```python
from build123d import *

# Parameters (mm, degrees)
ESQUISSE1_R        = 2
ESQUISSE1_W        = 5
ESQUISSE1_H        = 5
BOSS_EXTRU_1_DEPTH = 5
CONG_1_R           = 2


with BuildPart() as part:
    # Esquisse1 → Boss.-Extru.1 (new body)
    with BuildSketch(Plane.XY):
        with BuildLine():
            Line((-72.827296486, -27.9), (-72.827296486, 27.9))
            Line((-72.827296486, 27.9), (-25.4, 27.9))
            ThreePointArc((-25.4, 27.9), (-7.439487758, 20.460512242), (0, 2.5))
            Line((0, 2.5), (-10, 2.5))
            ThreePointArc((-10, 2.5), (-13.202056301, 3.42586604), (-15.41588754, 5.917721519))
            ThreePointArc((-15.41588754, 5.917721519), (-41.577296486, 0), (-15.41588754, -5.917721519))
            ThreePointArc((-15.41588754, -5.917721519), (-13.202056301, -3.42586604), (-10, -2.5))
            Line((-10, -2.5), (0, -2.5))
            ThreePointArc((0, -2.5), (-7.439487758, -20.460512242), (-25.4, -27.9))
            Line((-25.4, -27.9), (-72.827296486, -27.9))
        make_face()
        with Locations((-62.827296486, 0)):
            Circle(ESQUISSE1_R, mode=Mode.SUBTRACT)
        with Locations((-27.827296486, 20.4)):
            Rectangle(ESQUISSE1_W, ESQUISSE1_H, mode=Mode.SUBTRACT)
        Polygon((-9.245314739, 13.615063509), (-6.745314739, 9.284936491), (-11.075441758, 6.784936491), (-13.575441758, 11.115063509), align=None, mode=Mode.SUBTRACT)
        Polygon((-6.745314739, -9.284936491), (-9.245314739, -13.615063509), (-13.575441758, -11.115063509), (-11.075441758, -6.784936491), align=None, mode=Mode.SUBTRACT)
        with Locations((-27.827296486, -20.4)):
            Rectangle(ESQUISSE1_W, ESQUISSE1_H, mode=Mode.SUBTRACT)
        Polygon((-46.409278233, -13.615063509), (-48.909278233, -9.284936491), (-44.579151214, -6.784936491), (-42.079151214, -11.115063509), align=None, mode=Mode.SUBTRACT)
        Polygon((-48.909278233, 9.284936491), (-46.409278233, 13.615063509), (-42.079151214, 11.115063509), (-44.579151214, 6.784936491), align=None, mode=Mode.SUBTRACT)
    extrude(amount=BOSS_EXTRU_1_DEPTH)

    # Congé1
    cong_1_edges = [part.edges().sort_by_distance(p)[0] for p in [
        (0, 2.5, 2.5),
        (0, -2.5, 2.5),
    ]]
    fillet(cong_1_edges, radius=CONG_1_R)


solid = part.part
```
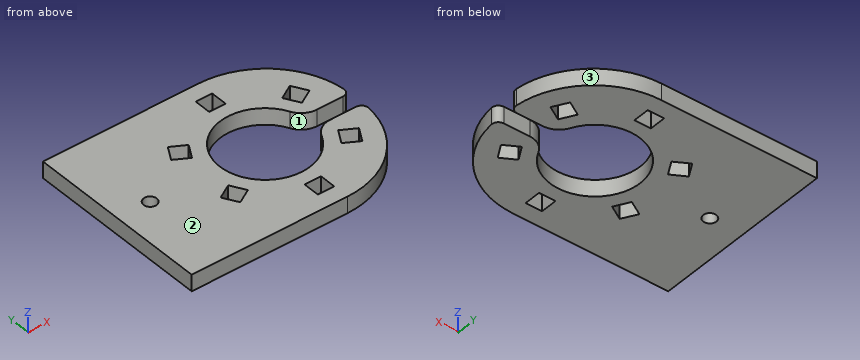
Source: CAD feature listing. Evaluate the final solid. Frame: model axes, mm. Face numbers are marked on the shaded views. Give positions to 0.01 mm unless a question says otherwise; leave off trailing zeros. Write each loop counter-clockwise with the first axis right and the second up, starting at its lowest first coordinate (ties: lowest second). Pieces come first, ordered by that corner, then holes.
1. First-contact query: pin 1 (3 mm diameter, centred on x = -62.83, y = 0, fed in from +Z); pin 2 (2.5 mm diameter, centred on x = -6, z = 2, fed in from +Y); pin 3 (1.5 mm diameter, centred on x = -7.5, z = 2, fed in from -Y); pin 4 (1.5 mm diameter, centred on y = -20, z = 2, fed in from +X). Flat tips, straight axial feed; report the tip coordinate or a pass-through.
2. Pull-direction query (X, two-part tool) for the marked faces 1, 2 and 3; classes: +X half, -X half, draft (parallel to the pull), parting line (faces both ways), or undercut.
3. Section query C-C (y = 24). Return the cut outline in (x, z), then the cut area to 3 significant figures.
4. Material intervals for line 1 along X through (y, z) = (12, 4.15); line 2 along Y through (x, z) = (-10, 2.9); line 3 along X through (y, z) = (-10, 2.3), sorted ascending.
5. Section query A-A (y = 0). Return the cut outline in (x, z), then the cut area to 3 significant figures.
6. Section query B-B (z = 2.45). Count the separate pieces of the cut face and the enclosed holes in it, then the cut area to 3 significant figures.
Output values:
1. pin 1: passes through
1. pin 2: stops at y = 20.27
1. pin 3: stops at y = -21.24
1. pin 4: stops at x = -6.31
2. face 1: undercut
2. face 2: draft
2. face 3: +X half
3. outline: (-72.83, 0) - (-11.88, 0) - (-11.88, 5) - (-72.83, 5) - close
3. area: 305 mm2
4. line 1: x = -72.83 to -47.34, -43.61 to -34.54, -21.11 to -12.04, -8.31 to -1.84
4. line 2: y = -22.7 to -13.18, -7.41 to -2.5, 2.5 to 7.41, 13.18 to 22.7
4. line 3: x = -72.83 to -48.5, -42.72 to -37.26, -18.39 to -12.93, -7.16 to -1.13
5. outline: (-72.83, 0) - (-64.83, 0) - (-64.83, 5) - (-72.83, 5) - close; (-60.83, 0) - (-41.58, 0) - (-41.58, 5) - (-60.83, 5) - close
5. area: 136 mm2
6. separate pieces: 1
6. enclosed holes: 7
6. area: 2,950 mm2
